Read the model definition and answer for the solid it produces. Units are mm, in the model's axes. A direction names the side the tool comes from. Give positions to 0.01 mm unless a question says otherwise; leave off trailing zeros. Write each loop counter-clockwise with the first axis right and the second up, starting at its lowest first coordinate (ties: lowest second). Pieces come first, ordered by that corner, then holes. Notation, with made-up numbers: M 83.25,40 L 126.25,40 A14 ccw 126.25,63 Z; hole C 20.5,13 d11. An arc over 180 degrees is marked long. Put each result on its own line as item: value.
from build123d import *

# Parameters (mm, degrees)
CYLINDER010_R     = 1.6
CYLINDER010_DEPTH = 5.32
CYLINDER008_R     = 1.6
CYLINDER008_DEPTH = 5.32
CYLINDER007_R     = 3.6
CYLINDER007_DEPTH = 6
CYLINDER006_R     = 3.6
CYLINDER006_DEPTH = 6
CUBE004_W         = 10
CUBE004_H         = 31.4
CUBE004_DEPTH     = 22.75
CYLINDER004_R     = 1.6
CYLINDER004_DEPTH = 5.32
CYLINDER002_R     = 1.6
CYLINDER002_DEPTH = 5.32
CYLINDER001_R     = 3.6
CYLINDER001_DEPTH = 6
CYLINDER_R        = 3.6
CYLINDER_DEPTH    = 6
CUBE003_W         = 10
CUBE003_H         = 31.4
CUBE003_DEPTH     = 22.75
CUBE002_W         = 3
CUBE002_H         = 0.4
CUBE002_DEPTH     = 23
CUBE001_W         = 19.4
CUBE001_H         = 19.4
CUBE001_DEPTH     = 23
CUBE_W            = 24.4
CUBE_H            = 24.4
CUBE_DEPTH        = 22


with BuildPart() as cylinder011:
    # cylinder011 → cylinder011 (revolve)
    with BuildSketch(Plane.XZ):
        Polygon((0, 0), (1.8, 0), (1.6, 1), (0, 1), align=None)
    revolve(axis=Axis((0, 0, 0), (0, 0, 1)))


with BuildPart() as union006:
    # cylinder010 → cylinder010 (new body)
    with BuildSketch(Plane.XY.offset(-0.01)):
        Circle(CYLINDER010_R)
    extrude(amount=CYLINDER010_DEPTH)

    # union006: union cylinder011
    add(cylinder011.part)


with BuildPart() as union006_1:
    # union006 placement: moved
    add(union006.part.moved(Location((17.2, 7, 0))))


with BuildPart() as cylinder009:
    # cylinder009 → cylinder009 (revolve)
    with BuildSketch(Plane.XZ):
        Polygon((0, 0), (1.8, 0), (1.6, 1), (0, 1), align=None)
    revolve(axis=Axis((0, 0, 0), (0, 0, 1)))


with BuildPart() as group003:
    # cylinder008 → cylinder008 (new body)
    with BuildSketch(Plane.XY.offset(-0.01)):
        Circle(CYLINDER008_R)
    extrude(amount=CYLINDER008_DEPTH)

    # union005: union cylinder009
    add(cylinder009.part)


with BuildPart() as group003_1:
    # union005 placement: moved
    add(group003.part.moved(Location((17.2, -7, 0))))

    # Group003: union union006
    add(union006_1.part)


with BuildPart() as cylinder007:
    # cylinder007 → cylinder007 (new body)
    with BuildSketch(Plane(origin=(17.2, 7, 0), x_dir=(1, 0, 0), z_dir=(0, 0, 1))):
        Circle(CYLINDER007_R)
    extrude(amount=CYLINDER007_DEPTH)


with BuildPart() as group002:
    # cylinder006 → cylinder006 (new body)
    with BuildSketch(Plane(origin=(17.2, -7, 0), x_dir=(1, 0, 0), z_dir=(0, 0, 1))):
        Circle(CYLINDER006_R)
    extrude(amount=CYLINDER006_DEPTH)

    # Group002: union cylinder007
    add(cylinder007.part)


with BuildPart() as difference002:
    # cube004 → cube004 (new body)
    with BuildSketch(Plane(origin=(12.2, -15.7, 0), x_dir=(1, 0, 0), z_dir=(0, 0, 1))):
        with Locations((5, 15.7)):
            Rectangle(CUBE004_W, CUBE004_H)
    extrude(amount=CUBE004_DEPTH)

    # union004: union Group002
    add(group002.part)

    # difference002: cut Group003
    add(group003_1.part, mode=Mode.SUBTRACT)


with BuildPart() as cylinder005:
    # cylinder005 → cylinder005 (revolve)
    with BuildSketch(Plane.XZ):
        Polygon((0, 0), (1.8, 0), (1.6, 1), (0, 1), align=None)
    revolve(axis=Axis((0, 0, 0), (0, 0, 1)))


with BuildPart() as union003:
    # cylinder004 → cylinder004 (new body)
    with BuildSketch(Plane.XY.offset(-0.01)):
        Circle(CYLINDER004_R)
    extrude(amount=CYLINDER004_DEPTH)

    # union003: union cylinder005
    add(cylinder005.part)


with BuildPart() as union003_1:
    # union003 placement: moved
    add(union003.part.moved(Location((-17.2, 7, 0))))


with BuildPart() as cylinder003:
    # cylinder003 → cylinder003 (revolve)
    with BuildSketch(Plane.XZ):
        Polygon((0, 0), (1.8, 0), (1.6, 1), (0, 1), align=None)
    revolve(axis=Axis((0, 0, 0), (0, 0, 1)))


with BuildPart() as group001:
    # cylinder002 → cylinder002 (new body)
    with BuildSketch(Plane.XY.offset(-0.01)):
        Circle(CYLINDER002_R)
    extrude(amount=CYLINDER002_DEPTH)

    # union002: union cylinder003
    add(cylinder003.part)


with BuildPart() as group001_1:
    # union002 placement: moved
    add(group001.part.moved(Location((-17.2, -7, 0))))

    # Group001: union union003
    add(union003_1.part)


with BuildPart() as cylinder001:
    # cylinder001 → cylinder001 (new body)
    with BuildSketch(Plane(origin=(-17.2, 7, 0), x_dir=(1, 0, 0), z_dir=(0, 0, 1))):
        Circle(CYLINDER001_R)
    extrude(amount=CYLINDER001_DEPTH)


with BuildPart() as group:
    # cylinder → cylinder (new body)
    with BuildSketch(Plane(origin=(-17.2, -7, 0), x_dir=(1, 0, 0), z_dir=(0, 0, 1))):
        Circle(CYLINDER_R)
    extrude(amount=CYLINDER_DEPTH)

    # Group: union cylinder001
    add(cylinder001.part)


with BuildPart() as group004:
    # cube003 → cube003 (new body)
    with BuildSketch(Plane(origin=(-22.2, -15.7, 0), x_dir=(1, 0, 0), z_dir=(0, 0, 1))):
        with Locations((5, 15.7)):
            Rectangle(CUBE003_W, CUBE003_H)
    extrude(amount=CUBE003_DEPTH)

    # union001: union Group
    add(group.part)

    # difference001: cut Group001
    add(group001_1.part, mode=Mode.SUBTRACT)

    # Group004: union difference002
    add(difference002.part)


with BuildPart() as cube002:
    # cube002 → cube002 (new body)
    with BuildSketch(Plane(origin=(-1.5, 9.7, -11.5), x_dir=(1, 0, 0), z_dir=(0, 0, 1))):
        with Locations((1.5, 0.2)):
            Rectangle(CUBE002_W, CUBE002_H)
    extrude(amount=CUBE002_DEPTH)


with BuildPart() as union:
    # cube001 → cube001 (new body)
    with BuildSketch(Plane(origin=(-9.7, -9.7, -11.5), x_dir=(1, 0, 0), z_dir=(0, 0, 1))):
        with Locations((9.7, 9.7)):
            Rectangle(CUBE001_W, CUBE001_H)
    extrude(amount=CUBE001_DEPTH)

    # union: union cube002
    add(cube002.part)


with BuildPart() as union007:
    # cube → cube (new body)
    with BuildSketch(Plane(origin=(-12.2, -12.2, -11), x_dir=(1, 0, 0), z_dir=(0, 0, 1))):
        with Locations((12.2, 12.2)):
            Rectangle(CUBE_W, CUBE_H)
    extrude(amount=CUBE_DEPTH)

    # difference: cut union
    add(union.part, mode=Mode.SUBTRACT)


with BuildPart() as union007_1:
    # difference placement: moved
    add(union007.part.moved(Location((0, 0, 11.75))))

    # union007: union Group004
    add(group004.part)


solid = union007_1.part
(1) Section A-A on y = 3.5 is taken. Determine the outline of the cut face in (x, z).
Result:
outline: M -22.2,0 L -12.2,0 L -12.2,0.75 L -9.7,0.75 L -9.7,22.75 L -22.2,22.75 Z; M 9.7,0.75 L 12.2,0.75 L 12.2,0 L 22.2,0 L 22.2,22.75 L 9.7,22.75 Z
(2) For a pull along Y with two mould halves and no side action, classify faces 5 (the face through (-17, -15.7, 11)), 6 (the face through (-18.47, 6.03, 3.12)), 7 (the face through (11, 0, 0.75)) as +Y half, -Y half, draft (parallel to the pull), parting line (faces both ways), or undercut.
Result:
face 5: -Y half
face 6: undercut
face 7: draft
(3) Section D-D on x = -17.2 is taken. Determine the outline of the cut face in (y, z), and give its area (3 significant figures).
Result:
outline: M -15.7,0 L -8.8,0 L -8.6,1 L -8.6,5.31 L -5.4,5.31 L -5.4,1 L -5.2,0 L 5.2,0 L 5.4,1 L 5.4,5.31 L 8.6,5.31 L 8.6,1 L 8.8,0 L 15.7,0 L 15.7,22.75 L -15.7,22.75 Z
area: 680 mm²
(4) Which of the six approach directions +Z, -Z, +X, -X, +Y, -Y give full straight-line access (tool end or side, diameter ignored) to faces 1 (the face through (0, -12.2, 12)), 2 (the face through (22.2, 0, 11)), 3 (the face through (-18.47, -7.97, 3.12)), 4 (the face through (-6, 9.7, 12))?
Result:
face 1: +Z, -Z, -Y
face 2: +Z, -Z, +X, +Y, -Y
face 3: -Z
face 4: +Z, -Z
(5) Section C-C on z = 10.25 is taken. Determine the outline of the cut face in (x, y), and give its area (3 significant figures).
Result:
outline: M -22.2,-15.7 L -12.2,-15.7 L -12.2,-12.2 L 12.2,-12.2 L 12.2,-15.7 L 22.2,-15.7 L 22.2,15.7 L 12.2,15.7 L 12.2,12.2 L -12.2,12.2 L -12.2,15.7 L -22.2,15.7 Z; hole M -9.7,-9.7 L 9.7,-9.7 L 9.7,9.7 L 1.5,9.7 L 1.5,10.1 L -1.5,10.1 L -1.5,9.7 L -9.7,9.7 Z
area: 846 mm²
(6) Section B-B on x = 0.5 is taken. Determine the outline of the cut face in (y, z), and give its area (3 significant figures).
Result:
outline: M -12.2,0.75 L -9.7,0.75 L -9.7,22.75 L -12.2,22.75 Z; M 10.1,0.75 L 12.2,0.75 L 12.2,22.75 L 10.1,22.75 Z
area: 101 mm²
(7) Straight lines are drawn through the part: line 1 along Y through (x, z) = (-17.2, 3.1); line 2 along X through (y, z) = (10, 8.5); line 3 along Y through (x, z) = (-6.5, 2.75). For each, find the intervals that lie inside material, in ascending order. Write a range as from..to.
Result:
line 1: y = -15.7..-8.6, -5.4..5.4, 8.6..15.7
line 2: x = -22.2..-1.5, 1.5..22.2
line 3: y = -12.2..-9.7, 9.7..12.2
(8) Given pin 1 Ø0.9 at (x, z) = (0.5, 8) entering from -Y; pin 2 Ø2.5 at (x, y) = (17.5, -7) entering from -Z; pin 3 Ø5 at (x, z) = (-0.5, 4.5) entering from +Y, each flat-ended and moving along its own axis, determine where each tip first touches the part or whether it passes through.
Result:
pin 1: stops at y = -12.2
pin 2: stops at z = 5.31
pin 3: stops at y = 12.2
